Geometry: final body of the model. Coordinates: model frame, mm. A direction names the side the tool comes from. Give positions to 0.01 mm unless a question says otherwise; leave off trailing zeros. Order: outer loops, then holes, each group sorted by start corner. A loop starts at its lowest first (then second) coordinate and runs counter-clockwise, first axis right, second up. Notation, with made-up numbers: (38, 6) - (65, 6) arc R24 cw to (65, 17) - close; hole circle Ø8 at (27.25, 37.5). An arc over 180 degrees is marked (long way). Use one line per item in the form item = value.
from build123d import *

# Parameters (mm, degrees)
SKETCH_1_R      = 20
EXTRUDE_1_DEPTH = 5
SKETCH_2_R      = 20
SKETCH_2_W      = 10
SKETCH_2_H      = 40
EXTRUDE_2_DEPTH = 2.5
SKETCH_3_W      = 50
SKETCH_3_H      = 50
SKETCH_3_R      = 1.8
EXTRUDE_3_DEPTH = 2


with BuildPart() as part:
    # 草图1 → 凸台-拉伸1 (new body, symmetric)
    with BuildSketch(Plane.XY):
        Circle(SKETCH_1_R)
    extrude(amount=EXTRUDE_1_DEPTH, both=True)

    # 草图2 → 凸台-拉伸2 (add, symmetric)
    with BuildSketch(Plane.XY):
        Circle(SKETCH_2_R)
        with Locations((0, 20)):
            Rectangle(SKETCH_2_W, SKETCH_2_H)
    extrude(amount=EXTRUDE_2_DEPTH, both=True)

    # 草图3 → 凸台-拉伸3 (add)
    with BuildSketch(Plane(origin=(0, 40, 0), x_dir=(1, 0, 0), z_dir=(0, 1, 0))):
        Rectangle(SKETCH_3_W, SKETCH_3_H)
        with Locations((-18.4, 18.4)):
            Circle(SKETCH_3_R, mode=Mode.SUBTRACT)
        with Locations((18.4, 18.4)):
            Circle(SKETCH_3_R, mode=Mode.SUBTRACT)
        with Locations((18.4, -18.4)):
            Circle(SKETCH_3_R, mode=Mode.SUBTRACT)
        with Locations((-18.4, -18.4)):
            Circle(SKETCH_3_R, mode=Mode.SUBTRACT)
    extrude(amount=-EXTRUDE_3_DEPTH)


solid = part.part
(1) Cut plane D-D on y = 0. Output: boundary loops of the cut face in (x, z), plus the area to 3 significant figures.
Computed values:
outline = (-20, -5) - (20, -5) - (20, 5) - (-20, 5) - close
area = 400 mm²
(2) Pull-direction query (Y, two-part tool) for faces 5 (the face through (0, 40, 0)), 6 (the face through (-16.737, 39.014, -17.711)), 7 (the face through (-4.336, -19.524, 0.07)); classes: released by +Y, released by -Y, zero draft, split by the parting line, or undercut.
Computed values:
face_5 = released by +Y
face_6 = zero draft
face_7 = undercut
(3) Contact query for flat-ended pins moving along their axis: pin 1 Ø4 at (x, y) = (4.5, 9) entering from +Z; pin 2 Ø1.5 at (y, z) = (30.5, 0.5) entering from +X; pin 3 Ø4 at (y, z) = (33.5, 0) entering from -X. Output: stop coordinate, or through.
Computed values:
pin_1 = 5
pin_2 = 5
pin_3 = -5
(4) Ray query, line 1 along X through (y, z) = (38.85, 18.4); line 2 along Z through (x, y) = (10, 13). Return the intervals inside material, ascending.
Computed values:
line_1 = -25 to -20.2, -16.6 to 16.6, 20.2 to 25
line_2 = -5 to 5
(5) Cut plane A-A on z = 18.4. Output: boundary loops of the cut face in (x, y), plus the area to 3 significant figures.
Computed values:
outline = (-25, 38) - (-20.2, 38) - (-20.2, 40) - (-25, 40) - close; (-16.6, 38) - (16.6, 38) - (16.6, 40) - (-16.6, 40) - close; (20.2, 38) - (25, 38) - (25, 40) - (20.2, 40) - close
area = 85.6 mm²
(6) Cut plane C-C on x = -18.4. Output: boundary loops of the cut face in (y, z), plus the area to 3 significant figures.
Computed values:
outline = (-7.84, -5) - (7.84, -5) - (7.84, 5) - (-7.84, 5) - close; (38, -25) - (40, -25) - (40, -20.2) - (38, -20.2) - close; (38, -16.6) - (40, -16.6) - (40, 16.6) - (38, 16.6) - close; (38, 20.2) - (40, 20.2) - (40, 25) - (38, 25) - close
area = 242 mm²
(7) Cut plane B-B on x = 0. Output: boundary loops of the cut face in (y, z), plus the area to 3 significant figures.
Computed values:
outline = (-20, -5) - (20, -5) - (20, -2.5) - (38, -2.5) - (38, -25) - (40, -25) - (40, 25) - (38, 25) - (38, 2.5) - (20, 2.5) - (20, 5) - (-20, 5) - close
area = 590 mm²
(8) Reachability of faces 1 (the face through (0, 0, -5)), 2 (the face through (5, 29, 0)), 3 (the face through (0, 0, 5)), 4 (the face through (-5, 29, 0)) from +Z, -Z, +X, -X, +Y, -Y: full face, straight path, thin tool, end or side. Return the list, or none.
Computed values:
face_1 = -Z, +X, -X, -Y
face_2 = +Z, -Z, +X
face_3 = +Z, +X, -X, -Y
face_4 = +Z, -Z, -X
